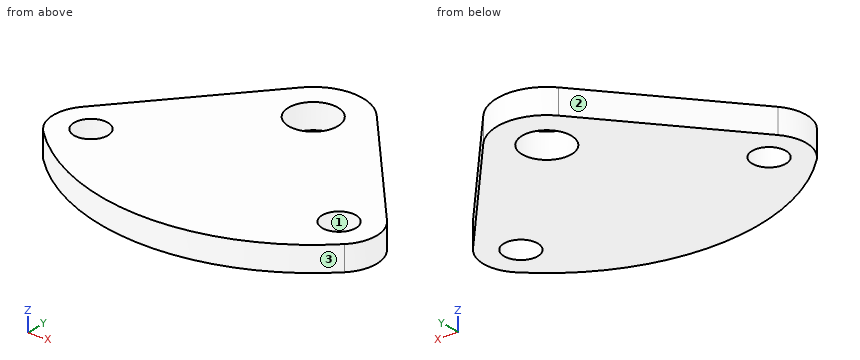
from build123d import *

# Parameters (mm, degrees)
F0_R     = 2.15265
F0_R_2   = 3.1369
F1_DEPTH = 3.175


with BuildPart() as f1:
    # F0 (on Top) → F1 (new body)
    with BuildSketch(Plane.XY):
        with BuildLine():
            Line((19.305298, -12.586502), (4.763557, 4.141088))
            ThreePointArc((4.763557, 4.141088), (0, 6.3119), (-4.763557, 4.141088))
            Line((-4.763557, 4.141088), (-19.305298, -12.586502))
            ThreePointArc((-19.305298, -12.586502), (-20.470666, -15.87722), (-19.078661, -19.078661))
            ThreePointArc((-19.078661, -19.078661), (0, -26.981301), (19.078661, -19.078661))
            ThreePointArc((19.078661, -19.078661), (20.470666, -15.87722), (19.305298, -12.586502))
        make_face()
        with Locations((-15.711065, -15.711065)):
            Circle(F0_R, mode=Mode.SUBTRACT)
        with Locations((15.711065, -15.711065)):
            Circle(F0_R, mode=Mode.SUBTRACT)
        Circle(F0_R_2, mode=Mode.SUBTRACT)
    extrude(amount=F1_DEPTH)


solid = f1.part
Design review of the part built by this model. Coordinates are the model's own, in mm. Face numbers are marked on the shaded views. Coordinates: 2 decimals unless noted, no trailing zeros. Write each loop counter-clockwise with the first axis right and the second up, starting at its lowest first coordinate (ties: lowest second). Pieces come first, ordered by that corner, then holes. Notation, with made-up numbers: (70.25, 59.5) - (77.25, 59.5) arc R13 ccw to (77.25, 79.5) - close; hole circle Ø8 at (89, -23). An arc over 180 degrees is marked (long way). One line per item, written item: value.
1) Mouldability with a two-part tool opening along X and no side actions: class the marked faces 1, 2 and 3 as +X half, -X half, draft (parallel to the pull), parting line (faces both ways), or undercut.
Answer sheet:
face 1: undercut
face 2: -X half
face 3: parting line
2) Add section C-C (y = 0). State the section outline as (x, z) points (3 decimals), plus the area to 3 significant figures.
Answer sheet:
outline: (-8.364, 0) - (-3.137, 0) - (-3.137, 3.175) - (-8.364, 3.175) - close; (3.137, 0) - (8.364, 0) - (8.364, 3.175) - (3.137, 3.175) - close
area: 33.2 mm2
3) Add section A-A (x = 0). State the section outline as (y, z) points (3 decimals), plus the area to 3 significant figures.
Answer sheet:
outline: (-26.981, 0) - (-3.137, 0) - (-3.137, 3.175) - (-26.981, 3.175) - close; (3.137, 0) - (6.312, 0) - (6.312, 3.175) - (3.137, 3.175) - close
area: 85.8 mm2
4) Insertion check: pin 1 (1 mm diameter, centred on x = 6, z = 1, fed in from +Y); pin 2 (3 mm diameter, centred on x = 10.5, y = 1, fed in from -Z). Each pin has a flat end and moves straight along its axis. Give the tip position at first contact, or say it passes through.
Answer sheet:
pin 1: stops at y = 3.29
pin 2: passes through
5) Add section D-D (y = -22.5). State the section outline as (x, z) points (3 decimals), plus the area to 3 significant figures.
Answer sheet:
outline: (-14.891, 0) - (14.891, 0) - (14.891, 3.175) - (-14.891, 3.175) - close
area: 94.6 mm2
6) To check wall thickness, follow probe 1 along X at (y, z) = (-17, 1.4); probe 2 along Y at (x, z) = (0, 2); probe 3 along X at (y, z) = (-2, 2.55). State the ranges of each line that lie inside material, in increasing order.
Answer sheet:
probe 1: x = -20.3 to -17.44, -13.99 to 13.99, 17.44 to 20.3
probe 2: y = -26.98 to -3.14, 3.14 to 6.31
probe 3: x = -10.1 to -2.42, 2.42 to 10.1
7) Add section B-B (z = 2.2). State the section outline as (x, y) points (1 decimal), plus the area to 3 significant figures.
Answer sheet:
outline: (-19.3, -12.6) arc R4.8 ccw to (-19.1, -19.1) arc R27 ccw to (19.1, -19.1) arc R4.8 ccw to (19.3, -12.6) - (4.8, 4.1) arc R6.3 ccw to (-4.8, 4.1) - close; hole circle Ø4.3 at (-15.7, -15.7); hole circle Ø6.3 at (0, 0); hole circle Ø4.3 at (15.7, -15.7)
area: 825 mm2
